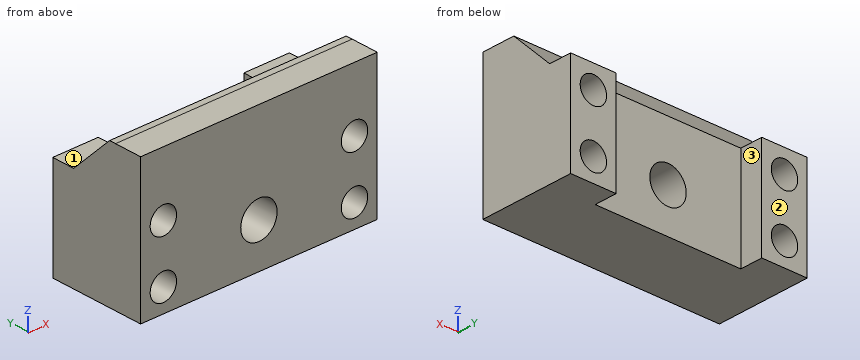
from build123d import *

# Parameters (mm, degrees)
SKETCH1_W            = 32
SKETCH1_H            = 23.261633661
SKETCH1_R            = 4
BOSS_EXTRUDE1_DEPTH  = 10
SKETCH3_W            = 10
SKETCH3_H            = 23.261633661
BOSS_EXTRUDE2_DEPTH  = 15
BOSS_EXTRUDE3_DEPTH  = 15
CUT_EXTRUDE1_DEPTH   = 61.230307985
M5_CLEARANCE_HOLE1_D = 5.8
CHAMFER1_SIZE        = 2
CHAMFER1_SIZE2       = 1.414213562
BOSS_EXTRUDE4_START  = 6
SKETCH9_W            = 52
SKETCH9_H            = 30.847420099
SKETCH9_R            = 2.9
SKETCH9_R_2          = 4
BOSS_EXTRUDE4_DEPTH  = 6


with BuildPart() as part:
    # Sketch1 → Boss-Extrude1 (new body)
    with BuildSketch(Plane(origin=(0, 0, 0), x_dir=(1, 0, 0), z_dir=(0, 1, 0))):
        with Locations((0, -2.06918317)):
            Rectangle(SKETCH1_W, SKETCH1_H)
        with Locations(Location((0, 0, 0), (0, 0, 270))):
            Circle(SKETCH1_R, mode=Mode.SUBTRACT)
    extrude(amount=-BOSS_EXTRUDE1_DEPTH)

    # Sketch3 → Boss-Extrude2 (add)
    with BuildSketch(Plane.XZ.offset(10)):
        with Locations((-21, 2.06918317)):
            Rectangle(SKETCH3_W, SKETCH3_H)
        with Locations((21, 2.06918317)):
            Rectangle(SKETCH3_W, SKETCH3_H)
    extrude(amount=-BOSS_EXTRUDE2_DEPTH)

    # Sketch5 → Boss-Extrude3 (add)
    with BuildSketch(Plane.XY.offset(13.7)):
        Polygon((16, 0), (-16, 0), (-16, 5), (-26, 5), (-26, -10), (26, -10), (26, 5), (16, 5), align=None)
    extrude(amount=BOSS_EXTRUDE3_DEPTH)

    # Sketch6 → Cut-Extrude1 (cut, through all)
    with BuildSketch(Plane.ZY.offset(26)):
        Polygon((12.7, 0), (22.7, -10), (28.7, -10), (28.7, 5), (12.7, 5), align=None)
    extrude(amount=-CUT_EXTRUDE1_DEPTH, mode=Mode.SUBTRACT)

    # M5 Clearance Hole1 (through all)
    with Locations(Plane(origin=(0, 5, 0), x_dir=(1, 0, 0), z_dir=(0, 1, 0))):
        with Locations((21, 4.561633661), (-21, 4.561633661), (-21, -7.7), (21, -7.7)):
            Hole(M5_CLEARANCE_HOLE1_D / 2)

    # Chamfer1
    chamfer1_edges = [part.edges().sort_by_distance(p)[0] for p in [
        (0, -10, 22.7),
    ]]
    chamfer1_side = [part.faces().sort_by_distance(p)[0] for p in [
        (0, -5, 17.7),
    ]]
    chamfer(chamfer1_edges, length=CHAMFER1_SIZE, length2=CHAMFER1_SIZE2, reference=chamfer1_side[0])

    # Sketch9 → Boss-Extrude4 (add)
    with BuildSketch(Plane.XZ.offset(10).offset(BOSS_EXTRUDE4_START)):
        with Locations((0, 5.862076389)):
            Rectangle(SKETCH9_W, SKETCH9_H)
        with Locations(Location((21, -4.561633661, 0), (0, 0, 90))):
            Circle(SKETCH9_R, mode=Mode.SUBTRACT)
        with Locations(Location((21, 7.7, 0), (0, 0, 90))):
            Circle(SKETCH9_R, mode=Mode.SUBTRACT)
        with Locations(Location((0, 0, 0), (0, 0, 90))):
            Circle(SKETCH9_R_2, mode=Mode.SUBTRACT)
        with Locations(Location((-21, -4.561633661, 0), (0, 0, 90))):
            Circle(SKETCH9_R, mode=Mode.SUBTRACT)
        with Locations(Location((-21, 7.7, 0), (0, 0, 90))):
            Circle(SKETCH9_R, mode=Mode.SUBTRACT)
    extrude(amount=-BOSS_EXTRUDE4_DEPTH)


solid = part.part
Input: part model. Units: mm. Frame: model coordinates. Face numbers are marked on the shaded views. A direction names the side the tool comes from. Coordinates: 2 decimals unless noted, no trailing zeros. Write each loop counter-clockwise with the first axis right and the second up, starting at its lowest first coordinate (ties: lowest second). Pieces come first, ordered by that corner, then holes. Notation, with made-up numbers: M -20.75,79.5 L 13.25,79.5 A23 cw 13.25,91.5 Z; hole C 17,86 d9. An arc over 180 degrees is marked long. Answer as a JSON object with one key per item and string values. Group by question number.
(1) Section B-B on x = 21. Output: boundary loops of the cut face in (y, z), plus the area to 3 significant figures.
(2) Section A-A on z = 7.7. Output: boundary loops of the cut face in (x, y), plus the area to 3 significant figures.
(3) Section D-D on y = -5. Output: boundary loops of the cut face in (x, z).
(4) Contact query for flat-ended pins moving along their axis: P1, Ø10, axis at x = 7.5, y = 1.5, coming from the +Z side; P2, Ø5, axis at x = 21, z = -4.56, coming from the +Y side; P3, Ø5.5, axis at x = 20, y = 3.5, coming from the +Z side; P4, Ø6.5, axis at x = 2, z = 2, coming from the +Y side. Output: stop coordinate, or through.
(5) Section C-C on y = 3. Output: boundary loops of the cut face in (x, z), plus the area to 3 significant figures.
(6) Ray query, line 1 along X through (y, z) = (1, -4.5); line 2 along Z through (x, y) = (21, 0.5); line 3 along X through (y, z) = (-10.5, -4.5). Return the intervals inside material, ascending. Write a range as [from, to].
(7) Set-up query: the marked faces 1, 2 and 3. Return all of +Z, -Z, +X, -X, +Y, -Y with unobstructed straight access to the full face (end or side cutting, diameter ignored); none if empty.
Result set:
{
 "1": {"outline": "M -16,-9.56 L 5,-9.56 L 5,-7.46 L -16,-7.46 Z; M -16,-1.66 L 5,-1.66 L 5,4.8 L -16,4.8 Z; M -16,10.6 L 5,10.6 L 5,12.7 L 0,12.7 L -8.59,21.29 L -16,21.29 Z", "area": "324 mm2"},
 "2": {"outline": "M -26,-16 L -23.9,-16 L -23.9,5 L -26,5 Z; M -18.1,-16 L 18.1,-16 L 18.1,5 L 16,5 L 16,0 L -16,0 L -16,5 L -18.1,5 Z; M 23.9,-16 L 26,-16 L 26,5 L 23.9,5 Z", "area": "688 mm2"},
 "3": {"outline": "M -26,-9.56 L 26,-9.56 L 26,17.7 L -26,17.7 Z; hole C -21,-4.56 d5.8; hole C -21,7.7 d5.8; hole C 0,0 d8; hole C 21,-4.56 d5.8; hole C 21,7.7 d5.8"},
 "4": {"P1": "stops at z = 16.2", "P2": "passes through", "P3": "stops at z = 12.7", "P4": "stops at y = 0"},
 "5": {"outline": "M -26,-9.56 L -16,-9.56 L -16,12.7 L -26,12.7 Z; M 16,-9.56 L 26,-9.56 L 26,12.7 L 16,12.7 Z; hole C -21,-4.56 d5.8; hole C -21,7.7 d5.8; hole C 21,-4.56 d5.8; hole C 21,7.7 d5.8", "area": "340 mm2"},
 "6": {"line 1": "x = [-26, -23.9], [-18.1, -16], [16, 18.1], [23.9, 26]", "line 2": "z = [-9.56, -7.46], [-1.66, 4.8], [10.6, 12.7]", "line 3": "x = [-26, -23.9], [-18.1, 18.1], [23.9, 26]"},
 "7": {"face 1": "+Z, +X, -X, +Y", "face 2": "+Z, -Z, +X, -X, +Y", "face 3": "+Z, -Z, +Y"}
}
